from build123d import *

# Parameters (mm, degrees)
F0_R     = 29.9
F1_DEPTH = 1.2
F2_R     = 29.9
F2_R_2   = 28.85
F3_DEPTH = 2
F4_R     = 2.5
F5_DEPTH = 3.2


with BuildPart() as f1:
    # F0 (on Top) → F1 (new body)
    with BuildSketch(Plane.XY):
        Circle(F0_R)
    extrude(amount=F1_DEPTH)

    # F2 (on face) → F3 (join)
    with BuildSketch(Plane.XY.offset(1.2)):
        Circle(F2_R)
        Circle(F2_R_2, mode=Mode.SUBTRACT)
    extrude(amount=F3_DEPTH)

    # F4 (on face) → F5 (cut)
    with BuildSketch(Plane.XY.offset(3.2)):
        with Locations((-11.251354, -26.56557)):
            Circle(F4_R)
    extrude(amount=-F5_DEPTH, mode=Mode.SUBTRACT)


solid = f1.part
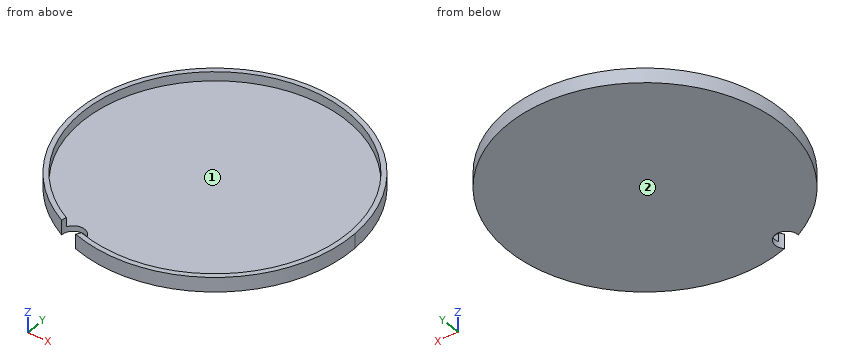
Work out the finished part from the listing and answer in its coordinate system (mm). Face numbers are marked on the shaded views. Round coordinates to 2 decimals unless told otherwise and drop trailing zeros. Loops run counter-clockwise (first coordinate to the right, second up) from the corner with the lowest first, then second, coordinate; pieces in that order, holes last. Notation, with made-up numbers: (0, 50.25) - (44, 50.25) arc R20 ccw to (44, 58.25) - close; hole circle Ø6 at (85, 71). An arc over 180 degrees is marked (long way). Use one line per item in the form item = value. Start each with the question number.
(1) Find section A-A on x = 0. Determine the outline of the cut face in (y, z), and give its area (3 significant figures).
(2) Flat-ended cylindrical pins translate along their axes: P1, Ø1.5, axis at x = -11.5, z = 2.5, coming from the +Y side; P2, Ø1.5, axis at x = -12.5, y = 20, coming from the +Z side; P3, Ø5, axis at x = -14, y = 11.5, coming from the -Z side. Find the tip coordinate at first contact, or state that the pin passes through.
(3) Consider line 1 (Z direction, x = 16, y = 20); line 2 (Y direction, x = 9, z = 2.5); line 3 (Y direction, x = -9, z = 0.4). Determine where each line is inside the solid, lowest interval first.
(4) Determine the mould class of the marked faces 1 and 2 for opening direction X: +X half, -X half, draft (parallel to the pull), parting line (faces both ways), or undercut.
(5) Find section B-B on y = -3. Determine the outline of the cut face in (x, z), and give its area (3 significant figures).
(6) Find section C-C on z = 2.2. Determine the outline of the cut face in (x, y).
Answer list:
q1.outline = (-29.9, 0) - (29.9, 0) - (29.9, 3.2) - (28.85, 3.2) - (28.85, 1.2) - (-28.85, 1.2) - (-28.85, 3.2) - (-29.9, 3.2) - close
q1.area = 76.0 mm^2
q2.P1 = 27.9
q2.P2 = 1.2
q2.P3 = 0
q3.line_1 = 0 to 1.2
q3.line_2 = -28.51 to -27.41, 27.41 to 28.51
q3.line_3 = -28.51 to -27.65, -25.48 to 28.51
q4.face_1 = undercut
q4.face_2 = draft
q5.outline = (-29.75, 0) - (29.75, 0) - (29.75, 3.2) - (28.69, 3.2) - (28.69, 1.2) - (-28.69, 1.2) - (-28.69, 3.2) - (-29.75, 3.2) - close
q5.area = 75.6 mm^2
q6.outline = (-13.75, -26.55) arc R2.5 cw to (-13.51, -25.49) arc R28.85 cw (long way) to (-8.91, -27.44) arc R2.5 cw to (-9.5, -28.35) arc R29.9 ccw (long way) to start
